```python
from build123d import *

# Parameters (mm, degrees)
ESQUISSE1_R        = 3.15
BOSS_EXTRU_1_DEPTH = 2
ESQUISSE2_R        = 15
BOSS_EXTRU_2_DEPTH = 3


with BuildPart() as part:
    # Esquisse1 → Boss.-Extru.1 (new body)
    with BuildSketch(Plane(origin=(0, 0, 0), x_dir=(1, 0, 0), z_dir=(0, 1, 0))):
        with BuildLine():
            Line((-25, -30), (25, -30))
            ThreePointArc((25, -30), (28.535533906, -28.535533906), (30, -25))
            Line((30, -25), (30, 25))
            ThreePointArc((30, 25), (28.535533906, 28.535533906), (25, 30))
            Line((25, 30), (-25, 30))
            ThreePointArc((-25, 30), (-28.535533906, 28.535533906), (-30, 25))
            Line((-30, 25), (-30, -25))
            ThreePointArc((-30, -25), (-28.535533906, -28.535533906), (-25, -30))
        make_face()
        with Locations((-24, 24)):
            Circle(ESQUISSE1_R, mode=Mode.SUBTRACT)
        with Locations((24, 24)):
            Circle(ESQUISSE1_R, mode=Mode.SUBTRACT)
        with Locations((24, -24)):
            Circle(ESQUISSE1_R, mode=Mode.SUBTRACT)
        with Locations((-24, -24)):
            Circle(ESQUISSE1_R, mode=Mode.SUBTRACT)
    extrude(amount=BOSS_EXTRU_1_DEPTH)

    # Esquisse2 → Boss.-Extru.2 (add)
    with BuildSketch(Plane(origin=(0, 2, 0), x_dir=(1, 0, 0), z_dir=(0, 1, 0))):
        Circle(ESQUISSE2_R)
    extrude(amount=BOSS_EXTRU_2_DEPTH)


solid = part.part
```
The listing builds one solid part. Answer for the finished solid, in the listing's coordinates (mm). A direction names the side the tool comes from. Round coordinates to 2 decimals unless told otherwise and drop trailing zeros. Loops run counter-clockwise (first coordinate to the right, second up) from the corner with the lowest first, then second, coordinate; pieces in that order, holes last.
Q1. Which of the six approach directions +Z, -Z, +X, -X, +Y, -Y give full straight-line access (tool end or side, diameter ignored) to faces 1 (the face through (0, 1, 30)), 2 (the face through (-7, 2, -14))?
Q2. Section D-D, the plane x = 0 is taken. Determine the outline of the cut face in (y, z), then the cut area to 3 significant figures.
Q3. Given pin 1 Ø3 at (x, z) = (-21.5, -10) entering from -Y; pin 2 Ø7 at (x, z) = (-24, -24) entering from +Y, each flat-ended and moving along its own axis, determine where each tip first touches the part or whether it passes through.
Q4. Section B-B, the plane x = -24 is taken. Determine the outline of the cut face in (y, z), then the cut area to 3 significant figures.
Q5. Section C-C, the plane y = 0.9 is taken. Determine the outline of the cut face in (x, z).
Q6. Find the intervals of material crossed by line 1 (Z direction, x = 24, y = 1.55); line 2 (X direction, y = 0.8, z = 25), in increasing order.
Q7. Section A-A, the plane z = -24 is taken. Determine the outline of the cut face in (x, y).
Q8. For a pull along X with two mould halves and no side action, classify faces 3 (the face through (-28, 1, -29)), 4 (the face through (23.317, 0.986, 27.075)), 5 (the face through (-14.985, 3.479, -0.66)) as released by +X, released by -X, zero draft, split by the parting line, or undercut.
Completed:
1. face 1: +Z, +X, -X, +Y, -Y
1. face 2: +Y
2. outline: (0, -30) - (2, -30) - (2, -15) - (5, -15) - (5, 15) - (2, 15) - (2, 30) - (0, 30) - close
2. area: 210 mm2
3. pin 1: stops at y = 0
3. pin 2: stops at y = 2
4. outline: (0, -30) - (2, -30) - (2, -27.15) - (0, -27.15) - close; (0, -20.85) - (2, -20.85) - (2, 20.85) - (0, 20.85) - close; (0, 27.15) - (2, 27.15) - (2, 30) - (0, 30) - close
4. area: 94.8 mm2
5. outline: (-30, -25) arc R5 ccw to (-25, -30) - (25, -30) arc R5 ccw to (30, -25) - (30, 25) arc R5 ccw to (25, 30) - (-25, 30) arc R5 ccw to (-30, 25) - close; hole circle Ø6.3 at (-24, -24); hole circle Ø6.3 at (-24, 24); hole circle Ø6.3 at (24, -24); hole circle Ø6.3 at (24, 24)
6. line 1: z = -30 to -27.15, -20.85 to 20.85, 27.15 to 30
6. line 2: x = -30 to -26.99, -21.01 to 21.01, 26.99 to 30
7. outline: (-30, 0) - (-27.15, 0) - (-27.15, 2) - (-30, 2) - close; (-20.85, 0) - (20.85, 0) - (20.85, 2) - (-20.85, 2) - close; (27.15, 0) - (30, 0) - (30, 2) - (27.15, 2) - close
8. face 3: released by -X
8. face 4: undercut
8. face 5: split by the parting line
